from build123d import *

# Parameters (mm, degrees)
SKETCH_R      = 2.5
PAD_DEPTH     = 5
SKETCH001_W   = 40
SKETCH001_H   = 50
SKETCH001_R   = 2.25
SKETCH001_R_2 = 2.5
PAD001_DEPTH  = 3
FILLET_R      = 10
PAD002_DEPTH  = 5
SKETCH003_R   = 1.25
SKETCH003_R_2 = 2.65
POCKET_DEPTH  = 8.001
FILLET001_R   = 1
FILLET002_R   = 1
FILLET003_R   = 1
FILLET004_R   = 3.5
FILLET005_R   = 1
FILLET006_R   = 1
FILLET007_R   = 1
FILLET008_R   = 1


with BuildPart() as part:
    # Sketch → Pad (new body)
    with BuildSketch(Plane.XY):
        with BuildLine():
            ThreePointArc((-10.842791, -1.853074), (-0.074616, -10.999747), (10.816654, -2))
            Line((7.228416, -2), (10.816654, -2))
            Line((7.228416, -2), (7.228416, 2))
            Line((10.816654, 2), (7.228416, 2))
            ThreePointArc((10.816654, 2), (-0.074616, 10.999747), (-10.842791, 1.853074))
            Line((-10.842791, 1.853074), (-7.26747, 1.853074))
            Line((-7.26747, -1.853074), (-7.26747, 1.853074))
            Line((-7.26747, -1.853074), (-10.842791, -1.853074))
        make_face()
        Circle(SKETCH_R, mode=Mode.SUBTRACT)
    extrude(amount=PAD_DEPTH)

    # Sketch001 → Pad001 (join)
    with BuildSketch(Plane.XY):
        with Locations((0, 5)):
            Rectangle(SKETCH001_W, SKETCH001_H)
        Circle(SKETCH001_R, mode=Mode.SUBTRACT)
        with Locations((0, 25)):
            Circle(SKETCH001_R_2, mode=Mode.SUBTRACT)
        with Locations((0, -15)):
            Circle(SKETCH001_R_2, mode=Mode.SUBTRACT)
    extrude(amount=-PAD001_DEPTH)

    # Fillet
    fillet_edges = [part.edges().sort_by_distance(p)[0] for p in [
        (20, -20, -1.5),
        (-20, -20, -1.5),
        (-20, 30, -1.5),
        (20, 30, -1.5),
    ]]
    fillet(fillet_edges, radius=FILLET_R)

    # Sketch002 (on Face2 of Fillet) → Pad002 (join)
    with BuildSketch(Plane.XY):
        with BuildLine():
            ThreePointArc((-4.371719, -12.7), (0, -20.126535), (4.371719, -12.7))
            Line((4.371719, -12.7), (-4.371719, -12.7))
        make_face()
        with BuildLine():
            ThreePointArc((4.439595, 12.7), (0, 20), (-4.439595, 12.7))
            Line((4.439595, 12.7), (-4.439595, 12.7))
        make_face()
    extrude(amount=PAD002_DEPTH)

    # Sketch003 (on Face30 of Pad002) → Pocket (cut, through all)
    with BuildSketch(Plane.XY.offset(5)):
        with Locations((0, 15)):
            Circle(SKETCH003_R)
        with Locations((0, -15)):
            Circle(SKETCH003_R_2)
    extrude(amount=-POCKET_DEPTH, mode=Mode.SUBTRACT)

    # Fillet001
    fillet001_edges = [part.edges().sort_by_distance(p)[0] for p in [
        (1.316245, -12.7, 2.5),
        (-1.316245, -12.7, 2.5),
    ]]
    fillet(fillet001_edges, radius=FILLET001_R)

    # Fillet002
    fillet002_edges = [part.edges().sort_by_distance(p)[0] for p in [
        (-4.371719, -12.7, 2.5),
    ]]
    fillet(fillet002_edges, radius=FILLET002_R)

    # Fillet003
    fillet003_edges = [part.edges().sort_by_distance(p)[0] for p in [
        (4.371719, -12.7, 2.5),
    ]]
    fillet(fillet003_edges, radius=FILLET003_R)

    # Fillet004
    fillet004_edges = [part.edges().sort_by_distance(p)[0] for p in [
        (-4.439595, 12.7, 2.5),
        (4.439595, 12.7, 2.5),
    ]]
    fillet(fillet004_edges, radius=FILLET004_R)

    # Fillet005
    fillet005_edges = [part.edges().sort_by_distance(p)[0] for p in [
        (-10.842791, 1.853074, 2.5),
        (-10.842791, -1.853074, 2.5),
    ]]
    fillet(fillet005_edges, radius=FILLET005_R)

    # Fillet006
    fillet006_edges = [part.edges().sort_by_distance(p)[0] for p in [
        (10.816654, 2, 2.5),
        (10.816654, -2, 2.5),
    ]]
    fillet(fillet006_edges, radius=FILLET006_R)

    # Fillet007
    fillet007_edges = [part.edges().sort_by_distance(p)[0] for p in [
        (-0.084509, -10.999675, 5),
    ]]
    fillet(fillet007_edges, radius=FILLET007_R)

    # Fillet008
    fillet008_edges = [part.edges().sort_by_distance(p)[0] for p in [
        (-0.084509, 10.999675, 5),
    ]]
    fillet(fillet008_edges, radius=FILLET008_R)


solid = part.part
The listing builds one solid part. Answer for the finished solid, in the listing's coordinates (mm). A direction names the side the tool comes from. Give positions to 0.01 mm unless a question says otherwise; leave off trailing zeros. Order: outer loops, then holes, each group sorted by start corner. A loop starts at its lowest first (then second) coordinate and runs counter-clockwise, first axis right, second up. Notation, with made-up numbers: (-1, -8.75) - (22, -8.75) arc R19 ccw to (22, 18.25) - close; hole circle Ø11 at (58, 81.25). An arc over 180 degrees is marked (long way). Use one line per item in the form item = value.
1) Find section C-C on x = 0. Give the number of separate pieces and of enclosed holes in the cut face, and give its area (3 significant figures).
Verdict:
separate_pieces = 5
enclosed_holes = 0
area = 219 mm^2
2) Find section B-B on z = 0.75. Determine the outline of the cut face in (x, y).
Verdict:
outline = (-10.54, -3.14) arc R11 ccw to (10.49, -3.3) arc R1 ccw to (9.54, -2) - (7.23, -2) - (7.23, 2) - (9.54, 2) arc R1 ccw to (10.49, 3.3) arc R11 ccw to (-10.54, 3.14) arc R1 ccw to (-9.58, 1.85) - (-7.27, 1.85) - (-7.27, -1.85) - (-9.58, -1.85) arc R1 ccw to start; (-4.67, -13.34) arc R5 ccw (long way) to (4.67, -13.34) arc R1 ccw to (3.74, -12.7) - (3.41, -12.7) arc R1 ccw to (2.48, -14.06) arc R2.65 cw (long way) to (-2.48, -14.06) arc R1 ccw to (-3.41, -12.7) - (-3.74, -12.7) arc R1 ccw to start; (-3, 19) arc R3.5 ccw to (-0.9, 12.7) - (0.9, 12.7) arc R3.5 ccw to (3, 19) arc R5 ccw to start; hole circle Ø5 at (0, 0); hole circle Ø2.5 at (0, 15)
3) Find section A-A on y = 0. Determine the outline of the cut face in (x, z), and give its area (3 significant figures).
Verdict:
outline = (-20, -3) - (-2.25, -3) - (-2.25, 0) - (-2.5, 0) - (-2.5, 5) - (-7.27, 5) - (-7.27, 0) - (-20, 0) - close; (2.25, -3) - (20, -3) - (20, 0) - (7.23, 0) - (7.23, 5) - (2.5, 5) - (2.5, 0) - (2.25, 0) - close
area = 154 mm^2
4) Find section D-D on y = 15. Determine the outline of the cut face in (x, z).
Verdict:
outline = (-20, -3) - (-1.25, -3) - (-1.25, 5) - (-4.19, 5) - (-4.19, 0) - (-20, 0) - close; (1.25, -3) - (20, -3) - (20, 0) - (4.19, 0) - (4.19, 5) - (1.25, 5) - close
5) Consider probe 1 along Y at (x, z) = (0, -1.8); probe 2 along Y at (x, z) = (0, 2.75); probe 3 along Y at (x, z) = (4, 4). Determine where each line is inside the solid, lowest interval first. Write a range as [from, to].
Verdict:
probe_1 = [-20, -17.65], [-12.35, -2.25], [2.25, 13.75], [16.25, 22.5], [27.5, 30]
probe_2 = [-20.13, -17.65], [-11, -2.5], [2.5, 11], [12.7, 13.75], [16.25, 20]
probe_3 = [-18.13, -12.74], [-10.25, 10.25], [14.58, 17.82]
6) Each of these flat-tipped pins is pushed along its axis until it touches: pin 1 (0.9 mm diameter, centred on x = -1, z = -2, fed in from -Y); pin 2 (8 mm diameter, centred on x = 0, y = 25, fed in from +Z); pin 3 (4 mm diameter, centred on x = -9, z = 4, fed in from +Y). Where does it stop, or does it pass through?
Verdict:
pin_1 = -20
pin_2 = 0
pin_3 = 8.49
7) The mould has two halves that part along X. Classify faces 1 (the cylindrical face through (0, 20, 2)), 2 (the cylindrical face through (-0.54, -2.44, 2.46)), 3 (the flat face through (0, 30, -1)): released by +X, released by -X, zero draft, split by the parting line, or undercut.
Verdict:
face_1 = split by the parting line
face_2 = undercut
face_3 = zero draft
8) For faces 4 (the cylindrical face through (-10.394, -2.266, 2.028)), 5 (the cylindrical face through (-0.29, 2.23, -1.48)), 6 (the cylindrical face through (0, 11, 2)), 7 (the cylindrical face through (10.353, -2.419, 2.028)), determine the directions among +Z, -Z, +X, -X, +Y, -Y from which every point of the face is accessible in a straight line to the end or side of a thin tool.
Verdict:
face_4 = +Z, -X
face_5 = +Z, -Z
face_6 = +Z
face_7 = +Z, +X
